For this review, take the finished solid that the model builds, in its own axes (mm). A direction names the side the tool comes from. Coordinates: 2 decimals unless noted, no trailing zeros. Order: outer loops, then holes, each group sorted by start corner. A loop starts at its lowest first (then second) coordinate and runs counter-clockwise, first axis right, second up. Notation, with made-up numbers: M 70,38 L 93,38 A24 ccw 93,54 Z; hole C -16.75,9 d6. An arc over 180 degrees is marked long. Use CSV: the item, a comma, the result in double quotes.
```python
from build123d import *

# Parameters (mm, degrees)
SKETCH1_W           = 127
SKETCH1_H           = 63.5
BOSS_EXTRUDE1_DEPTH = 5.08
SKETCH2_W           = 127
SKETCH2_H           = 63.5
SKETCH2_W_2         = 121.92
SKETCH2_H_2         = 58.42
BOSS_EXTRUDE3_DEPTH = 38.1
CUT_EXTRUDE1_REACH  = 150.411
SKETCH3_R           = 12.7
SKETCH3_R_2         = 2.159
FILLET3_R           = 5.08
FILLET4_R           = 2.54
CUT_EXTRUDE6_REACH  = 150.411
SKETCH4_R           = 6.35


with BuildPart() as part:
    # Sketch1 → Boss-Extrude1 (new body)
    with BuildSketch(Plane(origin=(0, 0, 0), x_dir=(1, 0, 0), z_dir=(0, 1, 0))):
        with Locations((63.5, 31.75)):
            Rectangle(SKETCH1_W, SKETCH1_H)
    extrude(amount=BOSS_EXTRUDE1_DEPTH)

    # Sketch2 → Boss-Extrude3 (add)
    with BuildSketch(Plane(origin=(0, 5.08, 0), x_dir=(1, 0, 0), z_dir=(0, 1, 0))):
        with Locations((63.5, 31.75)):
            Rectangle(SKETCH2_W, SKETCH2_H)
        with Locations((63.5, 31.75)):
            Rectangle(SKETCH2_W_2, SKETCH2_H_2, mode=Mode.SUBTRACT)
    extrude(amount=BOSS_EXTRUDE3_DEPTH)

    # Sketch3 → Cut-Extrude1 (cut, up to next)
    with BuildSketch(Plane.ZY, mode=Mode.PRIVATE) as cut_extrude1_sk1:
        with Locations((-31.75, 24.13)):
            Circle(SKETCH3_R)
    cut_extrude1_tool1 = extrude(cut_extrude1_sk1.sketch, amount=-CUT_EXTRUDE1_REACH, mode=Mode.PRIVATE) & part.part
    # Sketch3 → Cut-Extrude1 (cut, up to next)
    with BuildSketch(Plane.ZY, mode=Mode.PRIVATE) as cut_extrude1_sk2:
        with Locations((-46.9265, 35.3568)):
            Circle(SKETCH3_R_2)
    cut_extrude1_tool2 = extrude(cut_extrude1_sk2.sketch, amount=-CUT_EXTRUDE1_REACH, mode=Mode.PRIVATE) & part.part
    # Sketch3 → Cut-Extrude1 (cut, up to next)
    with BuildSketch(Plane.ZY, mode=Mode.PRIVATE) as cut_extrude1_sk3:
        with Locations((-16.5735, 35.3568)):
            Circle(SKETCH3_R_2)
    cut_extrude1_tool3 = extrude(cut_extrude1_sk3.sketch, amount=-CUT_EXTRUDE1_REACH, mode=Mode.PRIVATE) & part.part
    # Sketch3 → Cut-Extrude1 (cut, up to next)
    with BuildSketch(Plane.ZY, mode=Mode.PRIVATE) as cut_extrude1_sk4:
        with Locations((-46.9265, 12.9032)):
            Circle(SKETCH3_R_2)
    cut_extrude1_tool4 = extrude(cut_extrude1_sk4.sketch, amount=-CUT_EXTRUDE1_REACH, mode=Mode.PRIVATE) & part.part
    # Sketch3 → Cut-Extrude1 (cut, up to next)
    with BuildSketch(Plane.ZY, mode=Mode.PRIVATE) as cut_extrude1_sk5:
        with Locations((-16.5735, 12.9032)):
            Circle(SKETCH3_R_2)
    cut_extrude1_tool5 = extrude(cut_extrude1_sk5.sketch, amount=-CUT_EXTRUDE1_REACH, mode=Mode.PRIVATE) & part.part
    add(cut_extrude1_tool1.solids().sort_by_distance((0, 24.13, -31.75))[0], mode=Mode.SUBTRACT)
    add(cut_extrude1_tool2.solids().sort_by_distance((0, 35.3568, -46.9265))[0], mode=Mode.SUBTRACT)
    add(cut_extrude1_tool3.solids().sort_by_distance((0, 35.3568, -16.5735))[0], mode=Mode.SUBTRACT)
    add(cut_extrude1_tool4.solids().sort_by_distance((0, 12.9032, -46.9265))[0], mode=Mode.SUBTRACT)
    add(cut_extrude1_tool5.solids().sort_by_distance((0, 12.9032, -16.5735))[0], mode=Mode.SUBTRACT)

    # Fillet3
    fillet3_edges = [part.edges().sort_by_distance(p)[0] for p in [
        (0, 21.59, -63.5),
        (127, 21.59, -63.5),
        (127, 21.59, 0),
        (0, 21.59, 0),
    ]]
    fillet(fillet3_edges, radius=FILLET3_R)

    # Fillet4
    fillet4_edges = [part.edges().sort_by_distance(p)[0] for p in [
        (2.54, 24.13, -2.54),
        (124.46, 24.13, -2.54),
        (124.46, 24.13, -60.96),
        (2.54, 24.13, -60.96),
    ]]
    fillet(fillet4_edges, radius=FILLET4_R)

    # Sketch4 → Cut-Extrude6 (cut, up to next)
    with BuildSketch(Plane(origin=(127, 0, 0), x_dir=(0, 0, -1), z_dir=(1, 0, 0)), mode=Mode.PRIVATE) as cut_extrude6_sk1:
        with Locations((31.75, 24.13)):
            Circle(SKETCH4_R)
    cut_extrude6_tool1 = extrude(cut_extrude6_sk1.sketch, amount=-CUT_EXTRUDE6_REACH, mode=Mode.PRIVATE) & part.part
    add(cut_extrude6_tool1.solids().sort_by_distance((127, 24.13, -31.75))[0], mode=Mode.SUBTRACT)


solid = part.part
```
Item 1: Add section C-C on x = 39.5. State the section outline as (y, z) points, and give its area (3 significant figures).
Solutions:
outline,"M 0,-63.5 L 43.18,-63.5 L 43.18,-60.96 L 5.08,-60.96 L 5.08,-2.54 L 43.18,-2.54 L 43.18,0 L 0,0 Z"
area,"516 mm^2"
Item 2: Clearance check with flat-ended pins moving along their axes: pin 1 Ø2.5 at (y, z) = (35.36, -16.57) entering from -X; pin 2 Ø5 at (x, z) = (26.5, -16) entering from +Y. State where each tip first meets the part, or that it passes through.
Solutions:
pin 1,"x = 124.46"
pin 2,"y = 5.08"
Item 3: Add section B-B on z = -31.75. State the section outline as (x, y) points, and give its area (3 significant figures).
Solutions:
outline,"M 0,0 L 127,0 L 127,17.78 L 124.46,17.78 L 124.46,5.08 L 2.54,5.08 L 2.54,11.43 L 0,11.43 Z; M 0,36.83 L 2.54,36.83 L 2.54,43.18 L 0,43.18 Z; M 124.46,30.48 L 127,30.48 L 127,43.18 L 124.46,43.18 Z"
area,"742 mm^2"
Item 4: Add section A-A on y = 24.13. State the section outline as (x, z) points, and give its area (3 significant figures).
Solutions:
outline,"M 0,-58.42 A5.08 ccw 5.08,-63.5 L 121.92,-63.5 A5.08 ccw 127,-58.42 L 127,-38.1 L 124.46,-38.1 L 124.46,-58.42 A2.54 cw 121.92,-60.96 L 5.08,-60.96 A2.54 cw 2.54,-58.42 L 2.54,-44.45 L 0,-44.45 Z; M 0,-19.05 L 2.54,-19.05 L 2.54,-5.08 A2.54 cw 5.08,-2.54 L 121.92,-2.54 A2.54 cw 124.46,-5.08 L 124.46,-25.4 L 127,-25.4 L 127,-5.08 A5.08 ccw 121.92,0 L 5.08,0 A5.08 ccw 0,-5.08 Z"
area,"829 mm^2"
Item 5: Draft analysis for pull direction X (two halves, no side actions). For faces 1 (the face through (0, 12, -25)), 2 (the face through (63, 24, -60.96)), 3 (the face through (1.252, 32.713, -41.11)), state which applies: released by +X, released by -X, zero draft, split by the parting line, or undercut.
Solutions:
face 1,"released by -X"
face 2,"undercut"
face 3,"zero draft"
Item 6: To check wall thickness, follow line 1 along Y through (x, z) = (125.8, -31.75); line 2 along X through (y, z) = (7, -39.5); line 3 along Z through (x, y) = (86, 18). State the ranges of each line that lie inside material, in increasing order. Write a range as [from, to].
Solutions:
line 1,"[0, 17.78], [30.48, 43.18]"
line 2,"[0, 2.54], [124.46, 127]"
line 3,"[-63.5, -60.96], [-2.54, 0]"
Item 7: Add section D-D on y = 40. State the section outline as (x, z) points.
Solutions:
outline,"M 0,-58.42 A5.08 ccw 5.08,-63.5 L 121.92,-63.5 A5.08 ccw 127,-58.42 L 127,-5.08 A5.08 ccw 121.92,0 L 5.08,0 A5.08 ccw 0,-5.08 Z; hole M 2.54,-58.42 A2.54 ccw 5.08,-60.96 L 121.92,-60.96 A2.54 ccw 124.46,-58.42 L 124.46,-5.08 A2.54 ccw 121.92,-2.54 L 5.08,-2.54 A2.54 ccw 2.54,-5.08 Z"
Item 8: For faces 4 (the face through (127, 16, -31)), 5 (the face through (3.304, 24.397, -60.236)), 6 (the face through (1.25, 33.25, -47.39)), list the 3-axis set-ups (+Z, -Z, +X, -X, +Y, -Y) from which the entire face can be reached by the end or side of a thin tool; tool diameter is ignored.
Solutions:
face 4,"+Z, -Z, +X, +Y, -Y"
face 5,"+Y"
face 6,"-X"
